Part print with two shaded views. Sizes in mm from the minimum x, y, z corner. Round coordinates to 2 decimals unless told otherwise and drop trailing zeros. Order: outer loops, then holes, each group sorted by start corner. A loop starts at its lowest first (then second) coordinate and runs counter-clockwise, first axis right, second up. Notation, with made-up numbers: (15.25, -36.5) - (65.25, -36.5) arc R16 cw to (65.25, -22.5) - close; hole circle Ø5 at (63.25, -36). An arc over 180 degrees is marked (long way). Use one line per item in the form item = value.
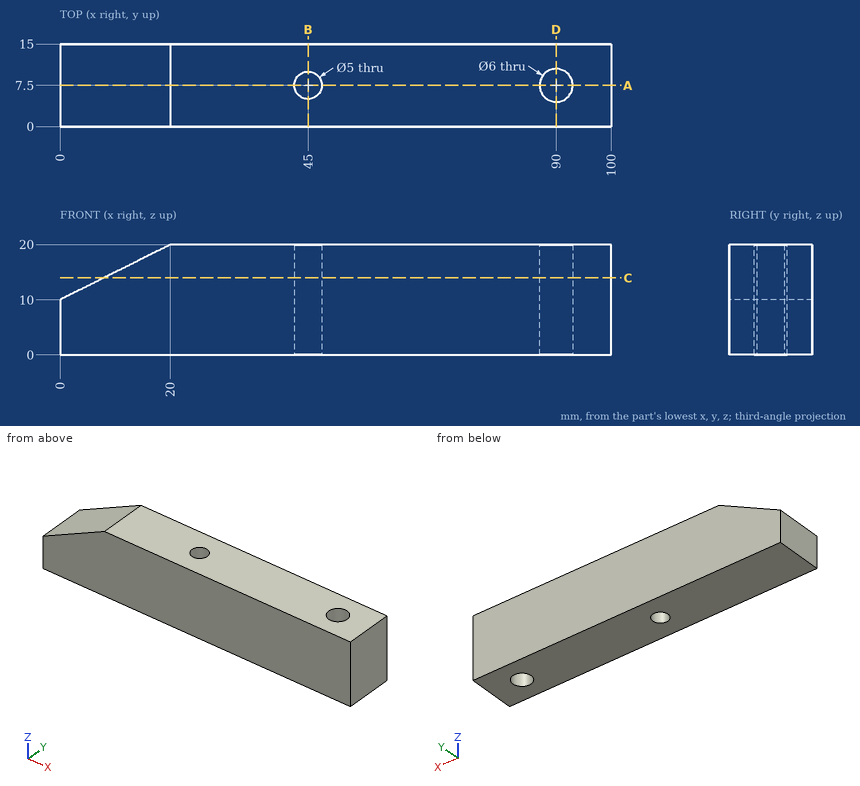
(1) Slice it at B-B on x = 45. Give the cut face in (y, z), then the cut area to 3 significant figures.
Report:
outline = (0, 0) - (5, 0) - (5, 20) - (0, 20) - close; (10, 0) - (15, 0) - (15, 20) - (10, 20) - close
area = 200 mm2
(2) Probe probe 1 along X at (y, z) = (7.75, 1.5); probe 2 along Y at (x, z) = (45, 9.25); probe 3 along Y at (x, z) = (90, 4.75). List the from-to ranges inside material, lowest first. Write a range as [from, to].
Report:
probe_1 = [0, 42.51], [47.49, 87.01], [92.99, 100]
probe_2 = [0, 5], [10, 15]
probe_3 = [0, 4.5], [10.5, 15]
(3) Slice it at C-C on z = 14. Give the cut face in (x, y), then the cut area to 3 significant figures.
Report:
outline = (8, 0) - (100, 0) - (100, 15) - (8, 15) - close; hole circle Ø5 at (45, 7.5); hole circle Ø6 at (90, 7.5)
area = 1,330 mm2
(4) Pin check, flat tips, straight feed: pin 1 (4.5 mm diameter, centred on x = 45, y = 7.5, fed in from -Z); pin 2 (1 mm diameter, centred on y = 3.5, z = 12.5, fed in from -X). Stop position of each tip, or through.
Report:
pin_1 = through
pin_2 = 4
(5) Slice it at A-A on y = 7.5. Give the cut face in (x, z).
Report:
outline = (0, 0) - (42.5, 0) - (42.5, 20) - (20, 20) - (0, 10) - close; (47.5, 0) - (87, 0) - (87, 20) - (47.5, 20) - close; (93, 0) - (100, 0) - (100, 20) - (93, 20) - close
(6) Slice it at D-D on x = 90. Give the cut face in (y, z), then the cut area to 3 significant figures.
Report:
outline = (0, 0) - (4.5, 0) - (4.5, 20) - (0, 20) - close; (10.5, 0) - (15, 0) - (15, 20) - (10.5, 20) - close
area = 180 mm2
